from build123d import *

# Parameters (mm, degrees)
BOSS_EXTRUDE1_DEPTH      = 7.587499938
BOSS_EXTRUDE1_DEPTH_BACK = 7.587499938
SKETCH1_R                = 6
SKETCH1_R_2              = 2
SKETCH2_R                = 2.749999953
CUT_EXTRUDE1_DEPTH       = 18.386219291


with BuildPart() as part:
    # Sketch1 → Boss-Extrude1 (new, two sides: drawn at the far end of the back side and taken through both)
    with BuildSketch(Plane(origin=(0, 0, 0), x_dir=(1, 0, 0), z_dir=(0, 1, 0)).offset(-BOSS_EXTRUDE1_DEPTH_BACK)):
        with Locations(Location((0, 0, 0), (0, 0, 270))):
            Circle(SKETCH1_R)
        with Locations(Location((0, 0, 0), (0, 0, 270))):
            Circle(SKETCH1_R_2, mode=Mode.SUBTRACT)
    extrude(amount=BOSS_EXTRUDE1_DEPTH + BOSS_EXTRUDE1_DEPTH_BACK)

    # Sketch2 → Cut-Extrude1 (cut, through all)
    with BuildSketch(Plane(origin=(0, 7.587499938, 0), x_dir=(1, 0, 0), z_dir=(0, 1, 0))):
        with Locations(Location((0, 0, 0), (0, 0, 270))):
            Circle(SKETCH2_R)
    extrude(amount=-CUT_EXTRUDE1_DEPTH, mode=Mode.SUBTRACT)

    # Cut-Extrude3 cone 1 section (through the dimple's axis) → Cut-Extrude3 (revolve, cut)
    with BuildSketch(Plane(origin=(0, 7.587499938, 0), x_dir=(0, 0, 1), z_dir=(1, 0, 0))):
        Polygon((0, 0), (3.249999953, 0), (0, 3.249999953), align=None)
    cut_extrude3 = revolve(axis=Axis((0, 7.587499938, 0), (0, -1, 0)), mode=Mode.SUBTRACT)

    # Mirror1: Cut-Extrude3 across plane
    add(cut_extrude3.mirror(Plane.ZX), mode=Mode.SUBTRACT)


solid = part.part
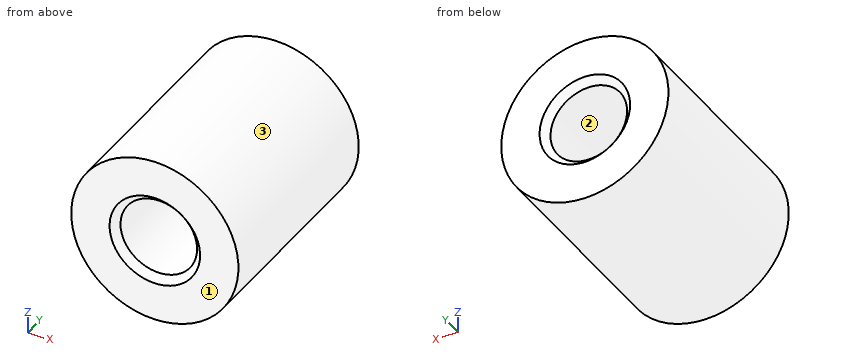
Verification items for the finished model (mm, model axes). Face numbers are marked on the shaded views. Coordinates: 2 decimals unless noted, no trailing zeros. Write each loop counter-clockwise with the first axis right and the second up, starting at its lowest first coordinate (ties: lowest second). Pieces come first, ordered by that corner, then holes. Notation, with made-up numbers: (-35, -3) - (6, -3) arc R16 cw to (6, 15) - close; hole circle Ø9 at (15, -15.75). An arc over 180 degrees is marked (long way). Answer as a JSON object with one key per item and string values.
(1) Cross-section at A-A on x = 0. Record the cut outline in (y, z).
Report:
{"outline": "(-7.59, -6) - (7.59, -6) - (7.59, -3.25) - (7.09, -2.75) - (-7.09, -2.75) - (-7.59, -3.25) - close; (-7.59, 3.25) - (-7.09, 2.75) - (7.09, 2.75) - (7.59, 3.25) - (7.59, 6) - (-7.59, 6) - close"}
(2) Gauge pin test, flat ends, axial feed: pin 1 Ø3 at (y, z) = (-2.5, 3.5) entering from -X; pin 2 Ø4 at (x, y) = (-3.5, -4.5) entering from +Z; pin 3 Ø5 at (x, y) = (-1, -5.5) entering from +Z; pin 4 Ø1 at (x, z) = (-2, -0.5) entering from -Y. Record the tip position at first contact, or that the pin passes through.
Report:
{"pin 1": "x = -5.66", "pin 2": "z = 5.81", "pin 3": "z = 6", "pin 4": "through"}
(3) Thickness scan on line 1 along X through (y, z) = (-3.25, 0); line 2 along X through (y, z) = (-2.5, 0.75); line 3 along Z through (x, y) = (0.5, 6.75). Record the ranges inside material, lowest first.
Report:
{"line 1": "-6 to -2.75, 2.75 to 6", "line 2": "-5.95 to -2.65, 2.65 to 5.95", "line 3": "-5.98 to -2.7, 2.7 to 5.98"}
(4) Cross-section at C-C on y = 6.25. Record the cut outline in (x, z).
Report:
{"outline": "circle Ø12 at (0, 0); hole circle Ø5.5 at (0, 0)"}
(5) Cross-section at D-D on z = -4. Record the cut outline in (x, y).
Report:
{"outline": "(-4.47, -7.59) - (4.47, -7.59) - (4.47, 7.59) - (-4.47, 7.59) - close"}
(6) Mould release check, pull along X, two halves, no side actions. Record for the marked faces 1, 2 and 3: pulls with the +X half, pulls with the -X half, needs draft (parallel to the pull), parting line crosses it, or undercut.
Report:
{"face 1": "needs draft", "face 2": "undercut", "face 3": "parting line crosses it"}
(7) Cross-section at B-B on z = 0. Record the cut outline in (x, y), plus the area to 3 significant figures.
Report:
{"outline": "(-6, -7.59) - (-3.25, -7.59) - (-2.75, -7.09) - (-2.75, 7.09) - (-3.25, 7.59) - (-6, 7.59) - close; (2.75, -7.09) - (3.25, -7.59) - (6, -7.59) - (6, 7.59) - (3.25, 7.59) - (2.75, 7.09) - close", "area": "98.1 mm^2"}
